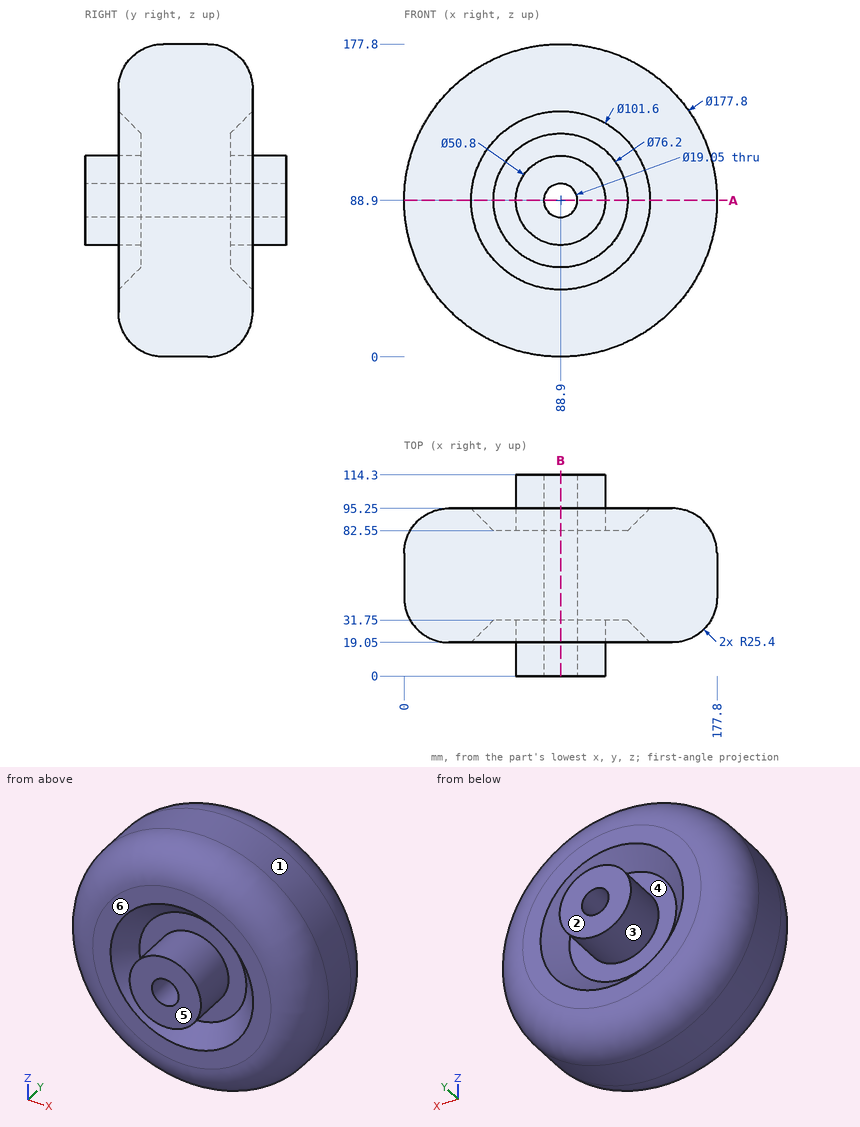
Study the drawing (mm; zero at the part's minimum x, y, z) and answer. A direction names the side the tool comes from. Coordinates: 2 decimals unless noted, no trailing zeros. Write each loop counter-clockwise with the first axis right and the second up, starting at its lowest first coordinate (ties: lowest second). Pieces come first, ordered by that corner, then holes. Notation, with made-up numbers: (17, 27.25) - (53, 27.25) arc R20 cw to (53, 49.25) - close; hole circle Ø6 at (44, 84). An arc over 180 degrees is marked (long way). One line per question, with ' | ' between items.
1) The mould has two halves that part along X. Classify the marked faces 1, 2 and 3: +X half, -X half, draft (parallel to the pull), parting line (faces both ways), or undercut.
Checks:
face 1: parting line | face 2: draft | face 3: undercut
2) Consider probe 1 along Z at (x, y) = (88, 51); probe 2 along X at (y, z) = (86, 67.5); probe 3 along Y at (x, z) = (153.5, 95.5). Determine where each line is inside the solid, lowest interval first. Write a range as [from, to].
Checks:
probe 1: [0, 79.42], [98.38, 177.8] | probe 2: [8.6, 53.28], [75.22, 102.58], [124.52, 169.2] | probe 3: [19.09, 95.21]
3) Find section B-B, the plane x = 88.9. Determine the outline of the cut face in (y, z) (3 decimals), and give its area (3 significant figures).
Checks:
outline: (0, 63.5) - (31.75, 63.5) - (31.75, 50.8) - (19.05, 38.1) - (19.05, 25.4) arc R25.4 ccw to (44.45, 0) - (69.85, 0) arc R25.4 ccw to (95.25, 25.4) - (95.25, 38.1) - (82.55, 50.8) - (82.55, 63.5) - (114.3, 63.5) - (114.3, 79.375) - (0, 79.375) - close; (0, 98.425) - (114.3, 98.425) - (114.3, 114.3) - (82.55, 114.3) - (82.55, 127) - (95.25, 139.7) - (95.25, 152.4) arc R25.4 ccw to (69.85, 177.8) - (44.45, 177.8) arc R25.4 ccw to (19.05, 152.4) - (19.05, 139.7) - (31.75, 127) - (31.75, 114.3) - (0, 114.3) - close | area: 11,800 mm2
4) Find section A-A, the plane z = 88.9. Determine the outline of the cut face in (x, y) (3 decimals).
Checks:
outline: (0, 44.45) arc R25.4 ccw to (25.4, 19.05) - (38.1, 19.05) - (50.8, 31.75) - (63.5, 31.75) - (63.5, 0) - (79.375, 0) - (79.375, 114.3) - (63.5, 114.3) - (63.5, 82.55) - (50.8, 82.55) - (38.1, 95.25) - (25.4, 95.25) arc R25.4 ccw to (0, 69.85) - close; (98.425, 0) - (114.3, 0) - (114.3, 31.75) - (127, 31.75) - (139.7, 19.05) - (152.4, 19.05) arc R25.4 ccw to (177.8, 44.45) - (177.8, 69.85) arc R25.4 ccw to (152.4, 95.25) - (139.7, 95.25) - (127, 82.55) - (114.3, 82.55) - (114.3, 114.3) - (98.425, 114.3) - close
5) Flat-ended cylindrical pins translate along their axes: P1, Ø12, axis at y = 93.5, z = 158.5, coming from the +X side; P2, Ø2, axis at y = 48, z = 145, coming from the +X side; P3, Ø2, axis at x = 50.5, z = 143.5, coming from the +Y side. Find the tip coordinate at first contact, or state that the pin passes through.
Checks:
P1: x = 135.03 | P2: x = 158.67 | P3: y = 95.15
6) For the marked faces 4, 5 and 6, determine the directions among +Z, -Z, +X, -X, +Y, -Y from which every point of the face is accessible in a straight line to the end or side of a thin tool.
Checks:
face 4: +Y | face 5: +Z, -Z, +X, -X, -Y | face 6: -Y
